Source: CAD feature listing. Evaluate the final solid. Frame: model axes, mm. Face numbers are marked on the shaded views. A direction names the side the tool comes from. Round coordinates to 2 decimals unless told otherwise and drop trailing zeros. Write each loop counter-clockwise with the first axis right and the second up, starting at its lowest first coordinate (ties: lowest second). Pieces come first, ordered by that corner, then holes.
Autodesk Inventor part; units mm, degrees
ref_plane "YZ Plane" through (0, 0, 0) normal (1, 0, 0) x (0, 1, 0)
ref_plane "XZ Plane" through (0, 0, 0) normal (0, 1, 0) x (-1, 0, 0)
ref_plane "XY Plane" through (0, 0, 0) normal (0, 0, 1) x (1, 0, 0)
sketch "Sketch1" plane through (0, 0, 0) normal (0, 1, 0) x (-1, 0, 0)
  circle A0 centre (0, 0) radius 30
  dimension "d0" = 60
extrude "Extrusion1" add sketch "Sketch1" against normal blind 6
sketch "Sketch2" plane through (0, 0, 0) normal (0, 1, 0) x (1, 0, 0)
  line L0 (-10, -18) -> (10, -18)
  line L1 (10, -32) -> (-10, -32)
  line L2 (-10, -18) -> (10, -32) construction
  line L3 (10, -18) -> (-10, -32) construction
  arc A0 (-7.5, -25) -> (-12.5, -25) centre (-10, -25) ccw
  arc A1 (12.5, -25) -> (7.5, -25) centre (10, -25) ccw
  line L4 (-12.5, -25) -> (12.5, -25)
  line L5 (-10, -32) -> (-10, -27.5)
  line L6 (-10, -25) -> (-10, -18)
  line L7 (10, -18) -> (10, -25)
  line L8 (10, -27.5) -> (10, -32)
  point P0 (0, 0)
  point P1 (0, -25)
  dimension "d3" = 20
  dimension "d4" = 25
  dimension "d5" = 14
  dimension "d6" = 5
  dimension "d7" = 5
revolve "Revolution1" cut sketch "Sketch2" angle 360 about axis through (-12.5, 0, 25) along (1, 0, 0)
sketch "Sketch3" plane through (0, -6, 0) normal (0, -1, 0) x (1, 0, 0)
  arc A0 (9.04, 28.6056) -> (-9.04, 28.6056) centre (0, 0) ccw
  line L0 (-9.04, 28.6056) -> (9.04, 28.6056)
  arc A1 (9.04, 28.6056) -> (-9.04, 28.6056) centre (0, 0) ccw
extrude "Extrusion2" cut sketch "Sketch3" against normal through all
fillet "Fillet1" radius 6 1 edges at (0, -6, -30)
pattern_circular "Circular Pattern1" count 4 over 360 about axis through (0, -10, 0) along (0, 1, 0) of "Revolution1"
sketch "Sketch4" plane through (0, -6, 0) normal (0, -1, 0) x (1, 0, 0)
  circle A0 centre (0, 0) radius 18
  dimension "d15" = 36
extrude "Extrusion3" cut sketch "Sketch4" against normal blind 2
sketch "Sketch5" plane through (0, -4, 0) normal (0, -1, 0) x (1, 0, 0)
  circle A0 centre (0, 0) radius 18
  line L0 (0, 0) -> (18, 0)
  line L1 (0, 0) -> (9.8995, 9.8995)
  line L2 (0, 0) -> (-9.8995, -9.8995)
  dimension "d19" = 45
  dimension "d20" = 14
  dimension "d21" = 14
  dimension "d22" = 180
hole "Hole1" at (9.8995, -4, 9.8995) at (-9.8995, -4, -9.8995) direction (0, 1, 0) diameter 4 end through all
properties part number "wheel_cover_in"
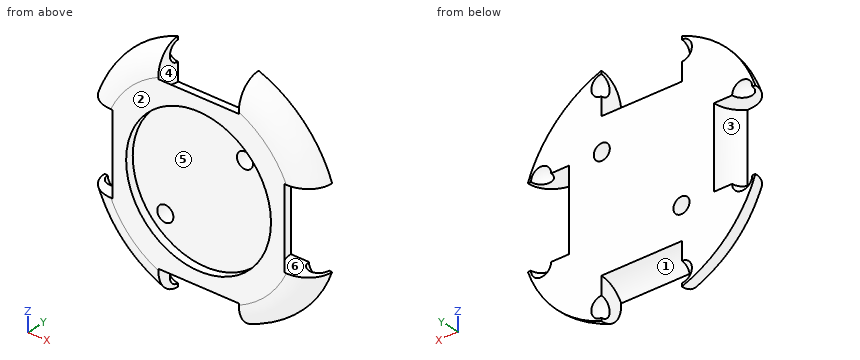
1) Section query B-B on z = 0. Return the cut outline in (x, y), then the cut area to 3 significant figures.
Taken from the geometry:
outline: (-21.39, -6) - (-18, -6) - (-18, -4) - (18, -4) - (18, -6) - (21.39, -6) arc R7 cw to (18, 0) - (-18, 0) arc R7 cw to start
area: 156 mm2
2) Section query A-A on x = 0. Return the cut outline in (y, z), then the cut area to 3 significant figures.
Taken from the geometry:
outline: (-6, -21.39) arc R7 cw to (0, -18) - (0, 18) arc R7 cw to (-6, 21.39) - (-6, 18) - (-4, 18) - (-4, -18) - (-6, -18) - close
area: 156 mm2
3) Material intervals for line 1 (Z direction, x = 21, y = -4.75); line 2 (Y direction, x = 3.5, z = 0); line 3 (Z direction, x = -20, y = -3.25), sorted ascending.
Taken from the geometry:
line 1: z = -18.01 to -10, 10 to 18.01
line 2: y = -4 to 0
line 3: z = -21.06 to -10, 10 to 21.06
4) Reachability of the marked faces 4, 5 and 6 from +Z, -Z, +X, -X, +Y, -Y: full face, straight path, thin tool, end or side. Return the list, or none.
Taken from the geometry:
face 4: +Z, +Y
face 5: -Y
face 6: +X, +Y
5) Pull-direction query (X, two-part tool) for the marked faces 1, 2 and 3; classes: released by +X, released by -X, zero draft, split by the parting line, or undercut.
Taken from the geometry:
face 1: undercut
face 2: zero draft
face 3: released by -X
6) Contact query for flat-ended pins moving along their axis: P1, Ø1.5, axis at x = -9, y = -1.5, coming from the -Z side; P2, Ø12, axis at x = 2, z = 2, coming from the -Y side; P3, Ø1.8, axis at x = 24, y = -3, coming from the +Z side; P4, Ø6.5, axis at x = -9.9, z = -9.9, coming from the +Y side. Output: stop coordinate, or through.
Taken from the geometry:
P1: stops at z = -18.37
P2: stops at y = -4
P3: stops at z = 18.08
P4: stops at y = 0
7) Section query C-C on y = -4.75. Return the cut outline in (x, z).
Taken from the geometry:
outline: (-25.8, -10) arc R27.67 ccw to (-10, -25.8) - (-10, -19.86) - (10, -19.86) - (10, -25.8) arc R27.67 ccw to (25.8, -10) - (19.86, -10) - (19.86, 10) - (25.8, 10) arc R27.67 ccw to (10, 25.8) - (10, 19.86) - (-10, 19.86) - (-10, 25.8) arc R27.67 ccw to (-25.8, 10) - (-19.86, 10) - (-19.86, -10) - close; hole circle Ø36 at (0, 0)
